Study the drawing (mm; zero at the part's minimum x, y, z) and answer. Give positions to 0.01 mm unless a question says otherwise; leave off trailing zeros. Write each loop counter-clockwise with the first axis right and the second up, starting at its lowest first coordinate (ties: lowest second). Pieces come first, ordered by that corner, then holes. Notation, with made-up numbers: (-24.75, -7.75) - (16.25, -7.75) arc R16 cw to (16.25, 3.25) - close; hole circle Ø2 at (-35.75, 85.5). An arc over 180 degrees is marked (long way). Return JSON: item names as keys, results as strings.
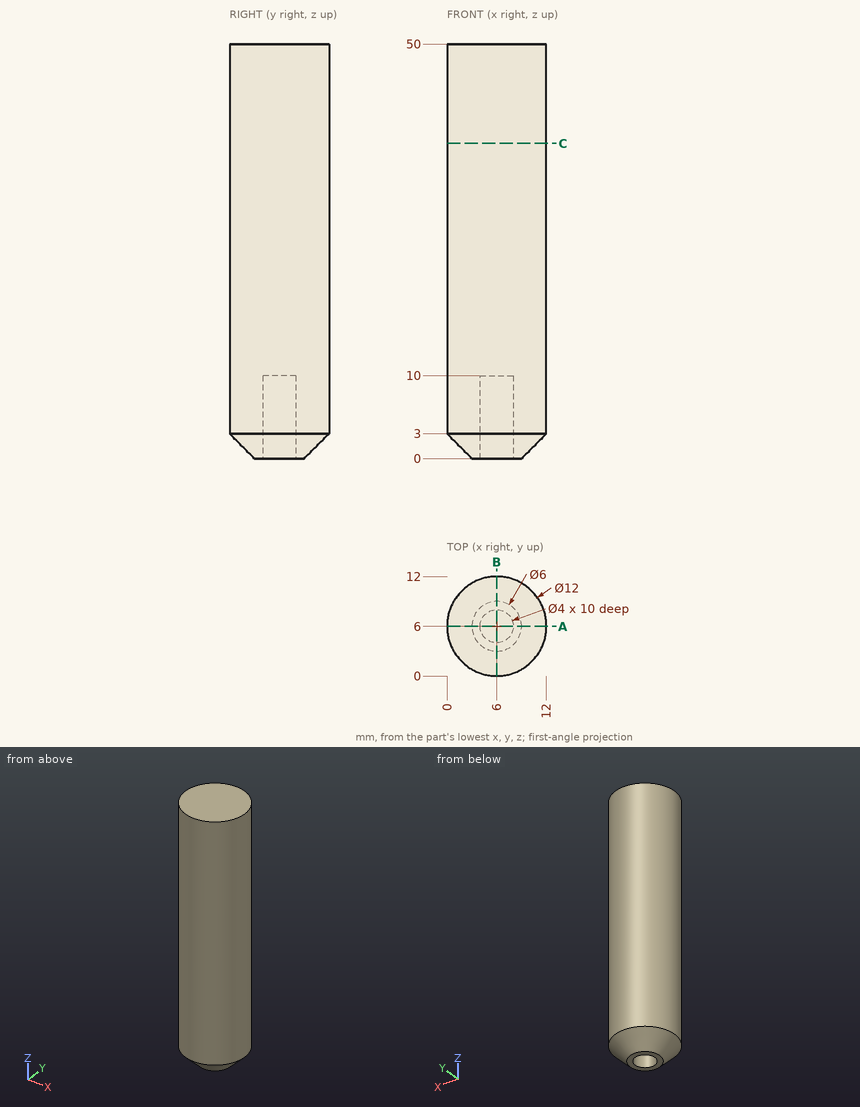
Item 1: Flat-ended cylindrical pins translate along their axes: P1, Ø1.5, axis at y = 5, z = 31.5, coming from the +X side; P2, Ø1.5, axis at x = 4, z = 31.5, coming from the -Y side; P3, Ø1, axis at x = 1, z = 21.5, coming from the -Y side. Find the tip coordinate at first contact, or state that the pin passes through.
Answer below:
{"P1": "stops at x = 11.99", "P2": "stops at y = 0.13", "P3": "stops at y = 2.03"}
Item 2: Consider L1, parallel to Y at x = 6, z = 4.75; L2, parallel to Y at x = 6, z = 2.5; L3, parallel to X at y = 5.75, z = 25.5. Determine where each line is inside the solid, lowest interval first.
Answer below:
{"L1": "y = 0 to 4, 8 to 12", "L2": "y = 0.5 to 4, 8 to 11.5", "L3": "x = 0.01 to 11.99"}
Item 3: A cutting plane is placed at C-C on z = 38. Determine the outline of the cut face in (x, y), then the cut area to 3 significant figures.
Answer below:
{"outline": "circle Ø12 at (6, 6)", "area": "113 mm²"}
Item 4: A cutting plane is placed at A-A on y = 6. Determine the outline of the cut face in (x, z), then the cut area to 3 significant figures.
Answer below:
{"outline": "(0, 3) - (3, 0) - (4, 0) - (4, 10) - (8, 10) - (8, 0) - (9, 0) - (12, 3) - (12, 50) - (0, 50) - close", "area": "551 mm²"}
